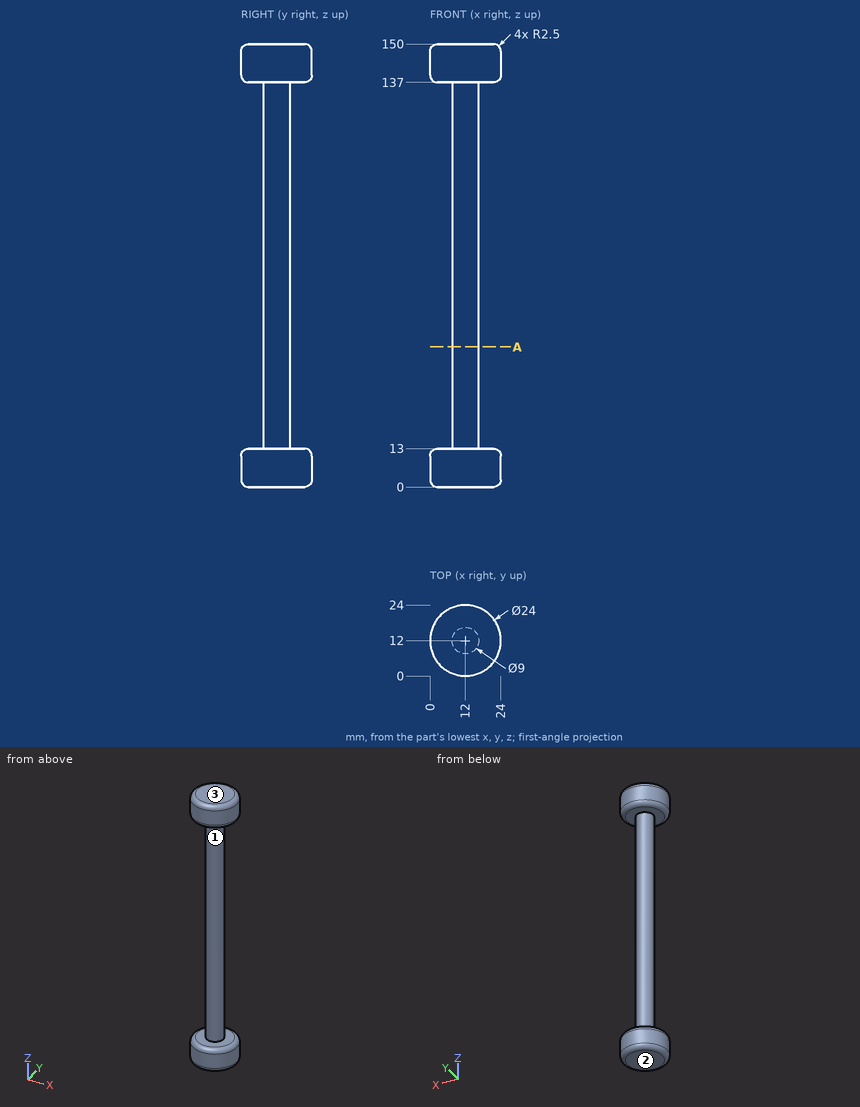
Answer from the drawing. Dimensions are ordinates in mm from the lowest x, y and z of the part. Round coordinates to 2 decimals unless told otherwise and drop trailing zeros. Write each loop counter-clockwise with the first axis right and the second up, starting at its lowest first coordinate (ties: lowest second). Pieces come first, ordered by that corner, then holes. Notation, with made-up numbers: (9.25, -8) -> (32.25, -8) arc R14 ccw to (32.25, 4) -> close; hole circle Ø5 at (86, -20.5). An arc over 180 degrees is marked (long way). Answer in a Markdown table with one row per item. Add a question column.
1) Given P1, Ø1.5, axis at y = 18.5, z = 125, coming from the +X side; P2, Ø8, axis at x = 7.5, z = 40, coming from the +Y side; P3, Ø1.5, axis at x = 15.5, z = 123, coming from the -Y side; P4, Ø10, axis at x = 3, z = 57.5, coming from the -Y side, each flat-ended and moving along its own axis, determine where each tip first touches the part or whether it passes through.
2) Determine the mould class of the marked faces 1, 2 and 3 for opening direction Z: pulls with the +Z half, pulls with the -Z half, needs draft (parallel to the pull), parting line crosses it, or undercut.
3) Find section A-A, the plane z = 47.5. Determine the outline of the cut face in (x, y).
4) Consider line 1 (Z direction, x = 6.5, y = 19.5); line 2 (Y direction, x = 11.5, z = 79); line 3 (Z direction, x = 2.5, y = 18). Determine where each line is inside the solid, lowest interval first.
Findings below:
| question | item | result |
|---|---|---|
| 1 | P1 | through |
| 1 | P2 | y = 16.47 |
| 1 | P3 | y = 8.44 |
| 1 | P4 | y = 9.94 |
| 2 | face 1 | undercut |
| 2 | face 2 | pulls with the -Z half |
| 2 | face 3 | pulls with the +Z half |
| 3 | outline | circle Ø9 at (12, 12) |
| 4 | line 1 | 0 to 13, 137 to 150 |
| 4 | line 2 | 7.53 to 16.47 |
| 4 | line 3 | 0.7 to 12.3, 137.7 to 149.3 |
